```python
from build123d import *

# Parameters (mm, degrees)
F0_W     = 152
F0_H     = 80
F1_DEPTH = 27
F2_W     = 150
F2_H     = 78
F3_DEPTH = 25
F4_R     = 6
F5_DEPTH = 5
F6_W     = 15
F6_H     = 15
F7_DEPTH = 1


with BuildPart() as f1:
    # F0 (on Top) → F1 (new body)
    with BuildSketch(Plane.XY):
        Rectangle(F0_W, F0_H)
    extrude(amount=F1_DEPTH)

    # F2 (on face) → F3 (cut)
    with BuildSketch(Plane.XY.offset(27)):
        Rectangle(F2_W, F2_H)
    extrude(amount=-F3_DEPTH, mode=Mode.SUBTRACT)

    # F4 (on face) → F5 (cut)
    with BuildSketch(Plane.XY.offset(2)):
        Circle(F4_R)
    extrude(amount=-F5_DEPTH, mode=Mode.SUBTRACT)

    # F6 (on face) → F7 (cut)
    with BuildSketch(Plane(origin=(0, 40, 0), x_dir=(-1, 0, 0), z_dir=(0, 1, 0))):
        with Locations((0, 19.5)):
            Rectangle(F6_W, F6_H)
    extrude(amount=-F7_DEPTH, mode=Mode.SUBTRACT)


solid = f1.part
```
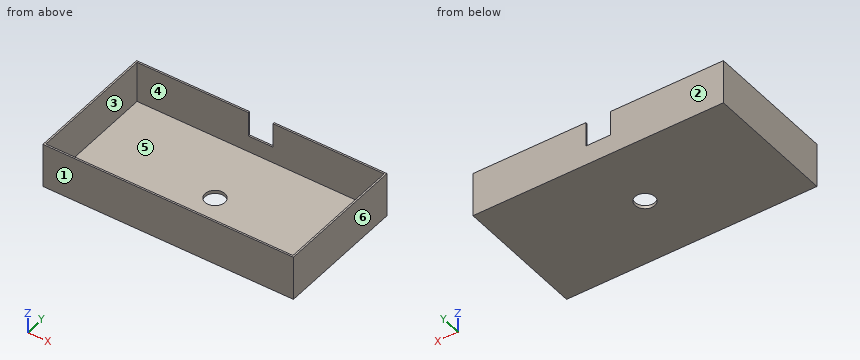
Could you check a few things on this model? Use its own coordinates, in mm. Face numbers are marked on the shaded views. A direction names the side the tool comes from. Round coordinates to 2 decimals unless told otherwise and drop trailing zeros. Loops run counter-clockwise (first coordinate to the right, second up) from the corner with the lowest first, then second, coordinate; pieces in that order, holes last. Notation, with made-up numbers: (47, 75.5) -> (63, 75.5) arc R21 cw to (63, 99.5) -> close; hole circle Ø4 at (-40, 17.5). An arc over 180 degrees is marked (long way). Put each result on its own line as item: value.
Q1. I want a section at B-B on x = 0. Write out the boundary of the cut face in (y, z).
Checks:
outline: (-40, 0) -> (-6, 0) -> (-6, 2) -> (-39, 2) -> (-39, 27) -> (-40, 27) -> close; (6, 0) -> (40, 0) -> (40, 12) -> (39, 12) -> (39, 2) -> (6, 2) -> close
Q2. Thinking about a two-plate mould opening in Y: for the marked faces 1, 2, 3 and 4, which applies, pulls with the +Y half, pulls with the -Y half, needs draft (parallel to the pull), parting line crosses it, or undercut?
Checks:
face 1: pulls with the -Y half
face 2: pulls with the +Y half
face 3: undercut
face 4: undercut
Q3. I want a section at A-A on y = 0. Write out the boundary of the cut face in (x, z).
Checks:
outline: (-76, 0) -> (-6, 0) -> (-6, 2) -> (-75, 2) -> (-75, 27) -> (-76, 27) -> close; (6, 0) -> (76, 0) -> (76, 27) -> (75, 27) -> (75, 2) -> (6, 2) -> close
Q4. I want a section at D-D on y = -19. Write out the boundary of the cut face in (x, z), and give its area (3 significant figures).
Checks:
outline: (-76, 0) -> (76, 0) -> (76, 27) -> (75, 27) -> (75, 2) -> (-75, 2) -> (-75, 27) -> (-76, 27) -> close
area: 354 mm2
Q5. Which directions (+Z, -Z, +X, -X, +Y, -Y) give clear straight access to the entire face, cutting with the end or side of a thin tool? Please do the marked faces 5 and 6.
Checks:
face 5: +Z
face 6: +Z, -Z, +X, +Y, -Y
Q6. I want a section at C-C on z = 9.5. Write out the boundary of the cut face in (x, y), and give its area (3 significant figures).
Checks:
outline: (-76, -40) -> (76, -40) -> (76, 40) -> (-76, 40) -> close; hole (-75, -39) -> (75, -39) -> (75, 39) -> (-75, 39) -> close
area: 460 mm2
Q7. Please list where these lines run through material, in increasing order: line 1 (X direction, y = -29.5, z = 17.75); line 2 (Y direction, x = 0, z = 1.4); line 3 (Y direction, x = 31.5, z = 6.5). Write a range as from..to.
Checks:
line 1: -76..-75, 75..76
line 2: -40..-6, 6..40
line 3: -40..-39, 39..40
Q8. For pin 1 Ø1.5 at (x, y) = (21, -11) entering from +Z, with a flat end and sliding along its axis, tell me the tip position at first contact or that it passes through.
Checks:
pin 1: z = 2
